Could you check a few things on this model? Use its own coordinates, in mm. A direction names the side the tool comes from. Round coordinates to 2 decimals unless told otherwise and drop trailing zeros. Loops run counter-clockwise (first coordinate to the right, second up) from the corner with the lowest first, then second, coordinate; pieces in that order, holes last. Notation, with made-up numbers: (54, 74) - (90, 74) arc R19 cw to (90, 95) - close; hole circle Ø7 at (89, 9). An arc over 180 degrees is marked (long way). Answer as CSV lines item,"result". Start each with the question number.
1) I'm going to push flat-ended pins straight in: pin 1 Ø5 at (x, y) = (-59, -116.64) entering from -Z; pin 2 Ø1.6 at (x, y) = (34.5, -88.5) entering from +Z (3 decimals); pin 3 Ø4.5 at (x, y) = (-46.47, -107.35) entering from +Z; pin 4 Ø1 at (x, z) = (-1, 0.5) entering from -Y. Where does each tip first touch, or does it pass through?
2) We'd pull the mould along Y, two halves only. Please class faces 3 (the face through (-3.992, -68.175, 1.972)), 4 (the face through (-21, -74, 4)), 5 (the face through (-46.52, 42.1, 1.97)): pulls with the +Y half, pulls with the -Y half, needs draft (parallel to the pull), parting line crosses it, or undercut.
3) Suppose I cut it at A-A, the plane x = -8. Write out the boundary of the cut face in (y, z), then the cut area to 3 significant figures.
4) Suppose I cut it at B-B, the plane z = 2.8. Count the separate pieces of the cut face and the enclosed holes in it, then the cut area to 3 significant figures.
5) Which directions (+Z, -Z, +X, -X, +Y, -Y) give clear straight access to the entire face, cutting with the end or side of a thin tool? Please do faces 1 (the face through (-45, -109, 1)), 2 (the face through (61, -77, 2)).
6) Please list where these lines run through material, in increasing order: line 1 along Y through (x, z) = (-95, 1.95); line 2 along Y through (x, z) = (-23, 1.9); line 3 along Y through (x, z) = (52.5, 2.2).
7) Suppose I cut it at C-C, the plane y = -27.5. Write out the boundary of the cut face in (x, z), then the cut area to 3 significant figures.
```python
from build123d import *

# Parameters (mm, degrees)
SKETCH1_R           = 83.5
SKETCH1_R_2         = 35
BOSS_EXTRUDE1_DEPTH = 4
CUT_EXTRUDE1_REACH  = 6
SKETCH2_R           = 1.6
SKETCH3_R           = 2.75
CUT_EXTRUDE2_DEPTH  = 3
BOSS_EXTRUDE2_DEPTH = 4
CUT_EXTRUDE3_REACH  = 6
SKETCH5_R           = 1.6
CUT_EXTRUDE4_DEPTH  = 2


with BuildPart() as part:
    # Sketch1 → Boss-Extrude1 (new body)
    with BuildSketch(Plane.XY):
        with Locations((-20.142161583, -37.124408079)):
            Circle(SKETCH1_R)
        with Locations((-20.142161583, -37.124408079)):
            Circle(SKETCH1_R_2, mode=Mode.SUBTRACT)
    extrude(amount=BOSS_EXTRUDE1_DEPTH)

    # Sketch2 → Cut-Extrude1 (cut, up to next)
    with BuildSketch(Plane.XY.offset(4), mode=Mode.PRIVATE) as cut_extrude1_sk1:
        with Locations((-51.182526114, 31.150739448)):
            Circle(SKETCH2_R)
    cut_extrude1_tool1 = extrude(cut_extrude1_sk1.sketch, amount=-CUT_EXTRUDE1_REACH, mode=Mode.PRIVATE) & part.part
    add(cut_extrude1_tool1.solids().sort_by_distance((-51.182526, 31.150739, 4))[0], mode=Mode.SUBTRACT)
    # Sketch2 → Cut-Extrude1 (cut, up to next)
    with BuildSketch(Plane.XY.offset(4), mode=Mode.PRIVATE) as cut_extrude1_sk2:
        with Locations((-22.691951254, 37.83223654)):
            Circle(SKETCH2_R)
    cut_extrude1_tool2 = extrude(cut_extrude1_sk2.sketch, amount=-CUT_EXTRUDE1_REACH, mode=Mode.PRIVATE) & part.part
    add(cut_extrude1_tool2.solids().sort_by_distance((-22.691951, 37.832237, 4))[0], mode=Mode.SUBTRACT)
    # Sketch2 → Cut-Extrude1 (cut, up to next)
    with BuildSketch(Plane.XY.offset(4), mode=Mode.PRIVATE) as cut_extrude1_sk3:
        with Locations((6.186805969, 33.102263974)):
            Circle(SKETCH2_R)
    cut_extrude1_tool3 = extrude(cut_extrude1_sk3.sketch, amount=-CUT_EXTRUDE1_REACH, mode=Mode.PRIVATE) & part.part
    add(cut_extrude1_tool3.solids().sort_by_distance((6.186806, 33.102264, 4))[0], mode=Mode.SUBTRACT)
    # Sketch2 → Cut-Extrude1 (cut, up to next)
    with BuildSketch(Plane.XY.offset(4), mode=Mode.PRIVATE) as cut_extrude1_sk4:
        with Locations((31.057216555, 17.680917193)):
            Circle(SKETCH2_R)
    cut_extrude1_tool4 = extrude(cut_extrude1_sk4.sketch, amount=-CUT_EXTRUDE1_REACH, mode=Mode.PRIVATE) & part.part
    add(cut_extrude1_tool4.solids().sort_by_distance((31.057217, 17.680917, 4))[0], mode=Mode.SUBTRACT)
    # Sketch2 → Cut-Extrude1 (cut, up to next)
    with BuildSketch(Plane.XY.offset(4), mode=Mode.PRIVATE) as cut_extrude1_sk5:
        with Locations((48.132985943, -6.084043548)):
            Circle(SKETCH2_R)
    cut_extrude1_tool5 = extrude(cut_extrude1_sk5.sketch, amount=-CUT_EXTRUDE1_REACH, mode=Mode.PRIVATE) & part.part
    add(cut_extrude1_tool5.solids().sort_by_distance((48.132986, -6.084044, 4))[0], mode=Mode.SUBTRACT)
    # Sketch2 → Cut-Extrude1 (cut, up to next)
    with BuildSketch(Plane.XY.offset(4), mode=Mode.PRIVATE) as cut_extrude1_sk6:
        with Locations((54.814483036, -34.574618408)):
            Circle(SKETCH2_R)
    cut_extrude1_tool6 = extrude(cut_extrude1_sk6.sketch, amount=-CUT_EXTRUDE1_REACH, mode=Mode.PRIVATE) & part.part
    add(cut_extrude1_tool6.solids().sort_by_distance((54.814483, -34.574618, 4))[0], mode=Mode.SUBTRACT)
    # Sketch2 → Cut-Extrude1 (cut, up to next)
    with BuildSketch(Plane.XY.offset(4), mode=Mode.PRIVATE) as cut_extrude1_sk7:
        with Locations((50.084510469, -63.453375632)):
            Circle(SKETCH2_R)
    cut_extrude1_tool7 = extrude(cut_extrude1_sk7.sketch, amount=-CUT_EXTRUDE1_REACH, mode=Mode.PRIVATE) & part.part
    add(cut_extrude1_tool7.solids().sort_by_distance((50.08451, -63.453376, 4))[0], mode=Mode.SUBTRACT)
    # Sketch2 → Cut-Extrude1 (cut, up to next)
    with BuildSketch(Plane.XY.offset(4), mode=Mode.PRIVATE) as cut_extrude1_sk8:
        with Locations((34.663163689, -88.323786218)):
            Circle(SKETCH2_R)
    cut_extrude1_tool8 = extrude(cut_extrude1_sk8.sketch, amount=-CUT_EXTRUDE1_REACH, mode=Mode.PRIVATE) & part.part
    add(cut_extrude1_tool8.solids().sort_by_distance((34.663164, -88.323786, 4))[0], mode=Mode.SUBTRACT)
    # Sketch2 → Cut-Extrude1 (cut, up to next)
    with BuildSketch(Plane.XY.offset(4), mode=Mode.PRIVATE) as cut_extrude1_sk9:
        with Locations((10.898202947, -105.399555606)):
            Circle(SKETCH2_R)
    cut_extrude1_tool9 = extrude(cut_extrude1_sk9.sketch, amount=-CUT_EXTRUDE1_REACH, mode=Mode.PRIVATE) & part.part
    add(cut_extrude1_tool9.solids().sort_by_distance((10.898203, -105.399556, 4))[0], mode=Mode.SUBTRACT)
    # Sketch2 → Cut-Extrude1 (cut, up to next)
    with BuildSketch(Plane.XY.offset(4), mode=Mode.PRIVATE) as cut_extrude1_sk10:
        with Locations((-17.592371912, -112.081052699)):
            Circle(SKETCH2_R)
    cut_extrude1_tool10 = extrude(cut_extrude1_sk10.sketch, amount=-CUT_EXTRUDE1_REACH, mode=Mode.PRIVATE) & part.part
    add(cut_extrude1_tool10.solids().sort_by_distance((-17.592372, -112.081053, 4))[0], mode=Mode.SUBTRACT)
    # Sketch2 → Cut-Extrude1 (cut, up to next)
    with BuildSketch(Plane.XY.offset(4), mode=Mode.PRIVATE) as cut_extrude1_sk11:
        with Locations((-46.471129136, -107.351080132)):
            Circle(SKETCH2_R)
    cut_extrude1_tool11 = extrude(cut_extrude1_sk11.sketch, amount=-CUT_EXTRUDE1_REACH, mode=Mode.PRIVATE) & part.part
    add(cut_extrude1_tool11.solids().sort_by_distance((-46.471129, -107.35108, 4))[0], mode=Mode.SUBTRACT)
    # Sketch2 → Cut-Extrude1 (cut, up to next)
    with BuildSketch(Plane.XY.offset(4), mode=Mode.PRIVATE) as cut_extrude1_sk12:
        with Locations((-71.341539722, -91.929733352)):
            Circle(SKETCH2_R)
    cut_extrude1_tool12 = extrude(cut_extrude1_sk12.sketch, amount=-CUT_EXTRUDE1_REACH, mode=Mode.PRIVATE) & part.part
    add(cut_extrude1_tool12.solids().sort_by_distance((-71.34154, -91.929733, 4))[0], mode=Mode.SUBTRACT)
    # Sketch2 → Cut-Extrude1 (cut, up to next)
    with BuildSketch(Plane.XY.offset(4), mode=Mode.PRIVATE) as cut_extrude1_sk13:
        with Locations((-88.41730911, -68.16477261)):
            Circle(SKETCH2_R)
    cut_extrude1_tool13 = extrude(cut_extrude1_sk13.sketch, amount=-CUT_EXTRUDE1_REACH, mode=Mode.PRIVATE) & part.part
    add(cut_extrude1_tool13.solids().sort_by_distance((-88.417309, -68.164773, 4))[0], mode=Mode.SUBTRACT)
    # Sketch2 → Cut-Extrude1 (cut, up to next)
    with BuildSketch(Plane.XY.offset(4), mode=Mode.PRIVATE) as cut_extrude1_sk14:
        with Locations((-95.098806203, -39.67419775)):
            Circle(SKETCH2_R)
    cut_extrude1_tool14 = extrude(cut_extrude1_sk14.sketch, amount=-CUT_EXTRUDE1_REACH, mode=Mode.PRIVATE) & part.part
    add(cut_extrude1_tool14.solids().sort_by_distance((-95.098806, -39.674198, 4))[0], mode=Mode.SUBTRACT)
    # Sketch2 → Cut-Extrude1 (cut, up to next)
    with BuildSketch(Plane.XY.offset(4), mode=Mode.PRIVATE) as cut_extrude1_sk15:
        with Locations((-90.368833636, -10.795440527)):
            Circle(SKETCH2_R)
    cut_extrude1_tool15 = extrude(cut_extrude1_sk15.sketch, amount=-CUT_EXTRUDE1_REACH, mode=Mode.PRIVATE) & part.part
    add(cut_extrude1_tool15.solids().sort_by_distance((-90.368834, -10.795441, 4))[0], mode=Mode.SUBTRACT)
    # Sketch2 → Cut-Extrude1 (cut, up to next)
    with BuildSketch(Plane.XY.offset(4), mode=Mode.PRIVATE) as cut_extrude1_sk16:
        with Locations((-74.947486856, 14.074970059)):
            Circle(SKETCH2_R)
    cut_extrude1_tool16 = extrude(cut_extrude1_sk16.sketch, amount=-CUT_EXTRUDE1_REACH, mode=Mode.PRIVATE) & part.part
    add(cut_extrude1_tool16.solids().sort_by_distance((-74.947487, 14.07497, 4))[0], mode=Mode.SUBTRACT)

    # Sketch3 → Cut-Extrude2 (cut)
    with BuildSketch(Plane.XY.offset(4)):
        with Locations((-74.947486856, 14.074970059)):
            Circle(SKETCH3_R)
        with Locations((-51.182526114, 31.150739448)):
            Circle(SKETCH3_R)
        with Locations((-22.691951254, 37.83223654)):
            Circle(SKETCH3_R)
        with Locations((6.186805969, 33.102263974)):
            Circle(SKETCH3_R)
        with Locations((31.057216555, 17.680917193)):
            Circle(SKETCH3_R)
        with Locations((48.132985943, -6.084043548)):
            Circle(SKETCH3_R)
        with Locations((54.814483036, -34.574618408)):
            Circle(SKETCH3_R)
        with Locations((50.084510469, -63.453375632)):
            Circle(SKETCH3_R)
        with Locations((34.663163689, -88.323786218)):
            Circle(SKETCH3_R)
        with Locations((10.898202947, -105.399555606)):
            Circle(SKETCH3_R)
        with Locations((-17.592371912, -112.081052699)):
            Circle(SKETCH3_R)
        with Locations((-46.471129136, -107.351080132)):
            Circle(SKETCH3_R)
        with Locations((-71.341539722, -91.929733352)):
            Circle(SKETCH3_R)
        with Locations((-88.41730911, -68.16477261)):
            Circle(SKETCH3_R)
        with Locations((-95.098806203, -39.67419775)):
            Circle(SKETCH3_R)
        with Locations((-90.368833636, -10.795440527)):
            Circle(SKETCH3_R)
    extrude(amount=-CUT_EXTRUDE2_DEPTH, mode=Mode.SUBTRACT)

    # Sketch4 → Boss-Extrude2 (add)
    with BuildSketch(Plane.XY.offset(4)):
        with BuildLine():
            ThreePointArc((7.293076451, 41.739764483), (20.915373779, 46.878739421), (25.229420752, 32.973163323))
            ThreePointArc((25.229420752, 32.973163323), (16.524193527, 37.894445571), (7.293076451, 41.739764483))
        make_face()
        with BuildLine():
            ThreePointArc((58.722010979, -64.559646114), (54.876692066, -73.790763189), (49.955409818, -82.495990414))
            ThreePointArc((49.955409818, -82.495990414), (63.860985917, -78.181943442), (58.722010979, -64.559646114))
        make_face()
        with BuildLine():
            ThreePointArc((-47.577399618, -115.988580642), (-56.808516694, -112.143261729), (-65.513743918, -107.221979481))
            ThreePointArc((-65.513743918, -107.221979481), (-61.199696946, -121.127555579), (-47.577399618, -115.988580642))
        make_face()
        with BuildLine():
            ThreePointArc((-99.006334146, -9.689170044), (-95.161015233, -0.458052969), (-90.239732985, 8.247174256))
            ThreePointArc((-90.239732985, 8.247174256), (-104.145309084, 3.933127284), (-99.006334146, -9.689170044))
        make_face()
    extrude(amount=-BOSS_EXTRUDE2_DEPTH)

    # Sketch5 → Cut-Extrude3 (cut, up to next)
    with BuildSketch(Plane(origin=(0, 0, 0), x_dir=(-1, 0, 0), z_dir=(0, 0, -1)), mode=Mode.PRIVATE) as cut_extrude3_sk1:
        with Locations((59.00410682, -116.635408654)):
            Circle(SKETCH5_R)
    cut_extrude3_tool1 = extrude(cut_extrude3_sk1.sketch, amount=-CUT_EXTRUDE3_REACH, mode=Mode.PRIVATE) & part.part
    add(cut_extrude3_tool1.solids().sort_by_distance((-59.004107, -116.635409, 0))[0], mode=Mode.SUBTRACT)
    # Sketch5 → Cut-Extrude3 (cut, up to next)
    with BuildSketch(Plane(origin=(0, 0, 0), x_dir=(-1, 0, 0), z_dir=(0, 0, -1)), mode=Mode.PRIVATE) as cut_extrude3_sk2:
        with Locations((-59.368838992, -75.986353316)):
            Circle(SKETCH5_R)
    cut_extrude3_tool2 = extrude(cut_extrude3_sk2.sketch, amount=-CUT_EXTRUDE3_REACH, mode=Mode.PRIVATE) & part.part
    add(cut_extrude3_tool2.solids().sort_by_distance((59.368839, -75.986353, 0))[0], mode=Mode.SUBTRACT)
    # Sketch5 → Cut-Extrude3 (cut, up to next)
    with BuildSketch(Plane(origin=(0, 0, 0), x_dir=(-1, 0, 0), z_dir=(0, 0, -1)), mode=Mode.PRIVATE) as cut_extrude3_sk3:
        with Locations((-18.719783653, 42.386592496)):
            Circle(SKETCH5_R)
    cut_extrude3_tool3 = extrude(cut_extrude3_sk3.sketch, amount=-CUT_EXTRUDE3_REACH, mode=Mode.PRIVATE) & part.part
    add(cut_extrude3_tool3.solids().sort_by_distance((18.719784, 42.386592, 0))[0], mode=Mode.SUBTRACT)
    # Sketch5 → Cut-Extrude3 (cut, up to next)
    with BuildSketch(Plane(origin=(0, 0, 0), x_dir=(-1, 0, 0), z_dir=(0, 0, -1)), mode=Mode.PRIVATE) as cut_extrude3_sk4:
        with Locations((99.653162158, 1.737537157)):
            Circle(SKETCH5_R)
    cut_extrude3_tool4 = extrude(cut_extrude3_sk4.sketch, amount=-CUT_EXTRUDE3_REACH, mode=Mode.PRIVATE) & part.part
    add(cut_extrude3_tool4.solids().sort_by_distance((-99.653162, 1.737537, 0))[0], mode=Mode.SUBTRACT)

    # Sketch6 → Cut-Extrude4 (cut)
    with BuildSketch(Plane(origin=(0, 0, 0), x_dir=(-1, 0, 0), z_dir=(0, 0, -1))):
        Polygon((-56.101046154, -76.375621821), (-57.397826158, -73.350995957), (-60.665618996, -72.961727451), (-62.636631829, -75.59708481), (-61.339851825, -78.621710675), (-58.072058987, -79.01097918), align=None)
        Polygon((55.979480955, -117.932188658), (58.614838314, -119.903201492), (61.639464179, -118.606421488), (62.028732685, -115.33862865), (59.393375325, -113.367615816), (56.368749461, -114.664395821), align=None)
        Polygon((-19.109052159, 39.118799658), (-16.084426294, 40.415579662), (-15.695157789, 43.6833725), (-18.330515148, 45.654385334), (-21.355141012, 44.357605329), (-21.744409518, 41.089812492), align=None)
        Polygon((96.385369321, 2.126805663), (97.682149325, -0.897820202), (100.949942163, -1.287088707), (102.920954996, 1.348268652), (101.624174992, 4.372894516), (98.356382154, 4.762163022), align=None)
    extrude(amount=-CUT_EXTRUDE4_DEPTH, mode=Mode.SUBTRACT)


solid = part.part
```
Filled sheet:
1,pin 1,"z = 2"
1,pin 2,"through"
1,pin 3,"z = 1"
1,pin 4,"y = -118.52"
2,face 3,"undercut"
2,face 4,"needs draft"
2,face 5,"pulls with the +Y half"
3,outline,"(-119.74, 0) - (-69.95, 0) - (-69.95, 4) - (-119.74, 4) - close; (-4.3, 0) - (45.49, 0) - (45.49, 4) - (-4.3, 4) - close"
3,area,"398 mm²"
4,separate pieces,"1"
4,enclosed holes,"21"
4,area,"18,300 mm²"
5,face 1,"+Z"
5,face 2,"-Z"
6,line 1,"-74.12 to -42.42, -36.93 to 9.54"
6,line 2,"-120.58 to -72.01, -2.24 to 35.1, 40.56 to 46.33"
6,line 3,"-83.5 to -64.77, -62.14 to -36.06, -33.09 to 4.05"
7,outline,"(-103.09, 0) - (-53.79, 0) - (-53.79, 4) - (-103.09, 4) - close; (13.51, 0) - (62.8, 0) - (62.8, 4) - (13.51, 4) - close"
7,area,"394 mm²"
